Source: CAD feature listing. Evaluate the final solid. Frame: model axes, mm. A direction names the side the tool comes from. Give positions to 0.01 mm unless a question says otherwise; leave off trailing zeros. Order: outer loops, then holes, each group sorted by start corner. A loop starts at its lowest first (then second) coordinate and runs counter-clockwise, first axis right, second up. Notation, with made-up numbers: M -0.75,85 L 15.25,85 A34 ccw 15.25,124 Z; hole C 8.5,-11.5 d10. An arc over 180 degrees is marked long. Use CSV: the item, a comma, the result in double quotes. Start each with the question number.
1. Pin query (flat end, axial travel): P1, Ø3, axis at x = -206, y = 3.5, coming from the +Z side; P2, Ø2, axis at x = -164, z = 57, coming from the +Y side; P3, Ø5, axis at y = 4, z = 52.2, coming from the -X side. Return the tip coordinate at first contact, or that it passes through.
2. Section query C-C, the plane y = 4. State how many separate pieces and enclosed holes the cut face has, plus the area to 3 significant figures.
3. Section query B-B, the plane z = 63. Return the cut outline in (x, y).
4. Line query: line 1 along Z through (x, y) = (-172.5, 4); line 2 along X through (y, z) = (0, 52.5); line 3 along Z through (x, y) = (-238, 3.5). Output: solid intervals per line, ascending. Write a range as [from, to].
5. Section query A-A, the plane x = -170. Return the cut outline in (y, z), plus the area to 3 significant figures.
6. Reachability of faces 4 (the cylindrical face through (-153.364, 4.127, -55.077)), 5 (the flat face through (-157.651, 6.1, 49.6)), 6 (the flat face through (-157.651, 6.1, -49.6)), 7 (the cylindrical face through (-235, 4, -57)), 8 (the flat face through (-249.394, 4, 48)) from +Z, -Z, +X, -X, +Y, -Y: full face, straight path, thin tool, end or side. Return the list, or none.
7. Mould query, pull axis Y, two halves, no side actions, for faces 1 (the cylindrical face through (-153, 4, 57)), 2 (the flat face through (-192.029, 4, 48)), 3 (the cylindrical face through (-176.627, 4.127, -55.077)). Classes: released by +Y, released by -Y, zero draft, split by the parting line, or undercut.
from build123d import *

# Parameters (mm, degrees)
BOSS_EXTRUDE1_DEPTH      = 8
BOSS_EXTRUDE2_DEPTH      = 46.583974855
BOSS_EXTRUDE2_DEPTH_BACK = 46.58397486
SKETCH4_R                = 2.4
SKETCH6_W                = 20
SKETCH6_H                = 3
BOSS_EXTRUDE3_DEPTH      = 30
CUT_EXTRUDE2_DEPTH       = 233.497849452
CUT_EXTRUDE2_DEPTH_BACK  = 233.497849452
SKETCH7_R                = 2
SKETCH8_W                = 40
SKETCH8_H                = 3
CUT_EXTRUDE3_DEPTH       = 40
SKETCH9_R                = 2
CUT_EXTRUDE4_DEPTH       = 40
FILLET1_R                = 20
SKETCH17_R               = 1.5
CUT_EXTRUDE10_DEPTH      = 25
SCALE1_SCALE             = 1.5
SKETCH18_W               = 192.636116151
SKETCH18_H               = 297.519421562
CUT_EXTRUDE11_DEPTH      = 304.953519557
SKETCH19_W               = 5
SKETCH19_H               = 12
CUT_EXTRUDE12_DEPTH      = 56.25
SKETCH20_W               = 35
SKETCH20_H               = 20.748828486
SKETCH20_W_2             = 15.531607356
SKETCH20_H_2             = 16.854299174
CUT_EXTRUDE13_DEPTH      = 304.953519557
FILLET2_R                = 2
FILLET3_R                = 7
FILLET4_R                = 2
SCALE2_SCALE             = 0.8
SKETCH21_R               = 1.8
BOSS_EXTRUDE4_DEPTH      = 9.6
SKETCH22_R               = 2
CUT_EXTRUDE14_DEPTH      = 270.167443306
SKETCH23_W               = 3.17304631
SKETCH23_H               = 12
SKETCH23_W_2             = 2.864071414
CUT_EXTRUDE15_DEPTH      = 270.167443306
SKETCH25_W               = 3.467321183
SKETCH25_H               = 12
CUT_EXTRUDE17_DEPTH      = 270.167443306


with BuildPart() as part:
    # Sketch1 → Boss-Extrude1 (new body)
    with BuildSketch(Plane(origin=(0, 0, 0), x_dir=(1, 0, 0), z_dir=(0, 1, 0))):
        Polygon((-120, -37.5), (-120, -75), (0, -75), (0, 75), (-120, 75), (-120, 37.5), (-220, 37.5), (-220, -37.5), align=None)
    extrude(amount=BOSS_EXTRUDE1_DEPTH)

    # Sketch4 → Boss-Extrude2 (add, two sides: drawn at the far end of the back side and taken through both)
    # profile 1 of 2: a face of its own
    with BuildSketch(Plane.ZY.offset(170).offset(-BOSS_EXTRUDE2_DEPTH_BACK)):
        with BuildLine():
            Line((37.5, 8), (43.5, 8))
            ThreePointArc((43.5, 8), (47.5, 4), (43.5, 0))
            Line((43.5, 0), (37.5, 0))
            Line((37.5, 0), (37.5, 8))
        make_face()
        with Locations((43.5, 4)):
            Circle(SKETCH4_R, mode=Mode.SUBTRACT)
    # profile 2 of 2: a face of its own
    with BuildSketch(Plane.ZY.offset(170).offset(-BOSS_EXTRUDE2_DEPTH_BACK)):
        with BuildLine():
            Line((-37.5, 0), (-43.5, 0))
            ThreePointArc((-43.5, 0), (-47.5, 4), (-43.5, 8))
            Line((-43.5, 8), (-37.5, 8))
            Line((-37.5, 8), (-37.5, 0))
        make_face()
        with Locations((-43.5, 4)):
            Circle(SKETCH4_R, mode=Mode.SUBTRACT)
    extrude(amount=BOSS_EXTRUDE2_DEPTH + BOSS_EXTRUDE2_DEPTH_BACK)

    # Sketch6 → Boss-Extrude3 (add)
    with BuildSketch(Plane(origin=(0, 0, 0), x_dir=(0, 0, -1), z_dir=(1, 0, 0))):
        with Locations((-50, 4)):
            Rectangle(SKETCH6_W, SKETCH6_H)
        with Locations((50, 4)):
            Rectangle(SKETCH6_W, SKETCH6_H)
    extrude(amount=BOSS_EXTRUDE3_DEPTH)

    # Sketch7 → Cut-Extrude2 (cut, two sides: drawn at the far end of the back side and taken through both)
    with BuildSketch(Plane(origin=(0, 5.5, 0), x_dir=(1, 0, 0), z_dir=(0, 1, 0)).offset(-CUT_EXTRUDE2_DEPTH_BACK)):
        with Locations(Location((22.5, 50, 0), (0, 0, 270))):
            Circle(SKETCH7_R)
        with Locations(Location((22.5, -50, 0), (0, 0, 270))):
            Circle(SKETCH7_R)
    extrude(amount=CUT_EXTRUDE2_DEPTH + CUT_EXTRUDE2_DEPTH_BACK, mode=Mode.SUBTRACT)

    # Sketch8 → Cut-Extrude3 (cut)
    with BuildSketch(Plane(origin=(0, 0, 0), x_dir=(0, 0, -1), z_dir=(1, 0, 0))):
        with Locations((0, 4)):
            Rectangle(SKETCH8_W, SKETCH8_H)
    extrude(amount=-CUT_EXTRUDE3_DEPTH, mode=Mode.SUBTRACT)

    # Sketch9 → Cut-Extrude4 (cut)
    with BuildSketch(Plane(origin=(0, 8, 0), x_dir=(1, 0, 0), z_dir=(0, 1, 0))):
        with Locations(Location((-32.5, 0, 0), (0, 0, 270))):
            Circle(SKETCH9_R)
    extrude(amount=-CUT_EXTRUDE4_DEPTH, mode=Mode.SUBTRACT)

    # Fillet1
    # the kernel refuses this fillet: 20 mm, written as the material it takes off along each edge
    with BuildSketch(Plane(origin=(-220, -27.947694226, -37.5), x_dir=(0, 0, 1), z_dir=(0, 1, 0))) as fillet1_piece_1:
        with BuildLine():
            CenterArc((11.17907769, 20), FILLET1_R, 236.01651728, 33.98348272)
            Line((0, 3.416025145), (-0.223581554, 3.084345648))
            ThreePointArc((-0.223581554, 3.084345648), (-0.4, 1.708012572), (-0.4, 0))
            Line((-0.4, 0), (0, -0.4))
            Line((0, -0.4), (11.17907769, -0.4))
            Line((11.17907769, -0.4), (11.17907769, 0))
        make_face()
    extrude(amount=63.895388452, mode=Mode.SUBTRACT)
    with BuildSketch(Plane(origin=(-220, -27.947694226, 37.5), x_dir=(1, 0, 0), z_dir=(0, 1, 0))) as fillet1_piece_2:
        with BuildLine():
            CenterArc((20, 11.17907769), FILLET1_R, 180, 33.98348272)
            Line((0, 11.17907769), (-0.4, 11.17907769))
            Line((-0.4, 11.17907769), (-0.4, 0))
            Line((-0.4, 0), (0, -0.4))
            ThreePointArc((0, -0.4), (1.708012572, -0.4), (3.084345648, -0.223581554))
            Line((3.084345648, -0.223581554), (3.416025145, 0))
        make_face()
    extrude(amount=63.895388452, mode=Mode.SUBTRACT)
    with BuildSketch(Plane(origin=(-120, -50, -75), x_dir=(1, 0, 0), z_dir=(0, 1, 0)), Plane(origin=(-120, -50, 75), x_dir=(0, 0, -1), z_dir=(0, 1, 0))) as fillet1_piece_3:
        with BuildLine():
            CenterArc((FILLET1_R, -FILLET1_R), FILLET1_R, 90, 90)
            Line((0, -FILLET1_R), (-FILLET1_R * 0.02, -FILLET1_R))
            Line((-FILLET1_R * 0.02, -FILLET1_R), (-FILLET1_R * 0.02, FILLET1_R * 0.02))
            Line((-FILLET1_R * 0.02, FILLET1_R * 0.02), (FILLET1_R, FILLET1_R * 0.02))
            Line((FILLET1_R, FILLET1_R * 0.02), (FILLET1_R, 0))
        make_face()
    extrude(amount=108, mode=Mode.SUBTRACT)

    # Sketch17 → Cut-Extrude10 (cut)
    with BuildSketch(Plane(origin=(0, 8, 0), x_dir=(1, 0, 0), z_dir=(0, 1, 0))):
        with Locations(Location((-75, 72.25, 0), (0, 0, 270))):
            Circle(SKETCH17_R)
        with Locations(Location((-25, 72.25, 0), (0, 0, 270))):
            Circle(SKETCH17_R)
        with Locations(Location((-25, -72.25, 0), (0, 0, 270))):
            Circle(SKETCH17_R)
        with Locations(Location((-75, -72.25, 0), (0, 0, 270))):
            Circle(SKETCH17_R)
    extrude(amount=-CUT_EXTRUDE10_DEPTH, mode=Mode.SUBTRACT)


with BuildPart() as part_1:
    # Scale1: scaled about (-95.774895805, 4, 0)
    add(part.part.scale(SCALE1_SCALE).moved(Location((47.887447902, -2, 0))))

    # Sketch18 → Cut-Extrude11 (cut, through all)
    with BuildSketch(Plane(origin=(0, 10, 0), x_dir=(1, 0, 0), z_dir=(0, 1, 0))):
        with Locations((64.205505977, 3.096142809)):
            Rectangle(SKETCH18_W, SKETCH18_H)
    extrude(amount=-CUT_EXTRUDE11_DEPTH, mode=Mode.SUBTRACT)

    # Sketch19 → Cut-Extrude12 (cut)
    with BuildSketch(Plane.XY.offset(112.5)):
        with Locations((-164.809163738, 4)):
            Rectangle(SKETCH19_W, SKETCH19_H)
    cut_extrude12 = extrude(amount=-CUT_EXTRUDE12_DEPTH, mode=Mode.SUBTRACT)

    # Mirror2: Cut-Extrude12 across plane
    add(cut_extrude12.mirror(Plane.XY), mode=Mode.SUBTRACT)

    # Sketch20 → Cut-Extrude13 (cut, through all)
    with BuildSketch(Plane(origin=(0, 10, 0), x_dir=(1, 0, 0), z_dir=(0, 1, 0))):
        with Locations((-223.406777288, -66.624414243)):
            Rectangle(SKETCH20_W, SKETCH20_H)
        with Locations((-143.974864216, -64.677149587)):
            Rectangle(SKETCH20_W_2, SKETCH20_H_2)
    cut_extrude13 = extrude(amount=-CUT_EXTRUDE13_DEPTH, mode=Mode.SUBTRACT)

    # Fillet2
    fillet2_edges = [part_1.edges().sort_by_distance(p)[0] for p in [
        (-162.309163738, 4, 56.25),
        (-167.309163738, 4, 56.25),
        (-205.906777288, 4, 56.25),
        (-240.906777288, 4, 56.25),
        (-151.740667894, 4, 56.25),
    ]]
    fillet(fillet2_edges, radius=FILLET2_R)

    # Mirror3: Cut-Extrude13 across plane
    add(cut_extrude13.mirror(Plane.XY), mode=Mode.SUBTRACT)

    # Fillet3
    fillet3_edges = [part_1.edges().sort_by_distance(p)[0] for p in [
        (-132.112552097, 4, 56.25),
        (-132.112552097, 4, -56.25),
    ]]
    fillet(fillet3_edges, radius=FILLET3_R)

    # Fillet4
    fillet4_edges = [part_1.edges().sort_by_distance(p)[0] for p in [
        (-162.309163738, 4, -56.25),
        (-167.309163738, 4, -56.25),
        (-240.906777288, 4, -56.25),
        (-205.906777288, 4, -56.25),
        (-151.740667894, 4, -56.25),
    ]]
    fillet(fillet4_edges, radius=FILLET4_R)


with BuildPart() as part_2:
    # Scale2: scaled about (-139.017271823, 4, 0)
    add(part_1.part.scale(SCALE2_SCALE).moved(Location((-27.803454365, 0.8, 0))))

    # Sketch21 → Boss-Extrude4 (add)
    with BuildSketch(Plane(origin=(0, 8.8, 0), x_dir=(1, 0, 0), z_dir=(0, 1, 0))):
        with Locations((-79.493496043, 86.7)):
            Circle(SKETCH21_R)
        with Locations((-79.493496043, -86.7)):
            Circle(SKETCH21_R)
    extrude(amount=-BOSS_EXTRUDE4_DEPTH)

    # Sketch22 → Cut-Extrude14 (cut, through all)
    with BuildSketch(Plane(origin=(0, 8.8, 0), x_dir=(1, 0, 0), z_dir=(0, 1, 0))):
        with Locations(Location((-78.432456753, 86.7, 0), (0, 0, 270))):
            Circle(SKETCH22_R)
        with Locations(Location((-78.432456753, -86.7, 0), (0, 0, 90))):
            Circle(SKETCH22_R)
    extrude(amount=-CUT_EXTRUDE14_DEPTH, mode=Mode.SUBTRACT)

    # Sketch23 → Cut-Extrude15 (cut, through all)
    with BuildSketch(Plane(origin=(0, 8.8, 0), x_dir=(1, 0, 0), z_dir=(0, 1, 0))):
        with Locations((-219.44235304, 51)):
            Rectangle(SKETCH23_W, SKETCH23_H)
        with Locations((-219.44235304, -51)):
            Rectangle(SKETCH23_W, SKETCH23_H)
        with Locations((-193.460911902, 51)):
            Rectangle(SKETCH23_W_2, SKETCH23_H)
        with Locations((-193.460911902, -51)):
            Rectangle(SKETCH23_W_2, SKETCH23_H)
    extrude(amount=-CUT_EXTRUDE15_DEPTH, mode=Mode.SUBTRACT)

    # Sketch25 → Cut-Extrude17 (cut, through all)
    with BuildSketch(Plane(origin=(0, 8.8, 0), x_dir=(1, 0, 0), z_dir=(0, 1, 0))):
        with Locations((-219.995215604, -51)):
            Rectangle(SKETCH25_W, SKETCH25_H)
        with Locations((-219.995215604, 51)):
            Rectangle(SKETCH25_W, SKETCH25_H)
    extrude(amount=-CUT_EXTRUDE17_DEPTH, mode=Mode.SUBTRACT)


solid = part_2.part
Result set:
1,P1,"z = 45"
1,P2,"y = 6.93"
1,P3,"x = -133.57"
2,separate pieces,"7"
2,enclosed holes,"2"
2,area,"25,700 mm2"
3,outline,"M -133.49,-0.8 L -53.49,-0.8 L -53.49,8.8 L -133.49,8.8 Z"
4,line 1,"[-57, -55.08], [-49.32, 49.32], [55.08, 57]"
4,line 2,"[-249.39, -221.73], [-192.03, -161.65], [-157.65, -149.2], [-133.49, -53.49]"
4,line 3,"[-56.97, -55.04], [-49.36, 49.36], [55.04, 56.97]"
5,outline,"M -0.8,-52.2 A4.8 ccw 8.8,-52.2 L 8.8,52.2 A4.8 ccw -0.8,52.2 Z; hole C 4,-52.2 d5.76; hole C 4,52.2 d5.76"
5,area,"1,020 mm2"
6,face 4,"-X"
6,face 5,"+Z, +Y, -Y"
6,face 6,"-Z, +Y, -Y"
6,face 7,"-Z, -X"
6,face 8,"+Z, -X, +Y, -Y"
7,face 1,"split by the parting line"
7,face 2,"zero draft"
7,face 3,"undercut"
